Check sheet for the drawn part. Datum: minimum x, y, z corner. Units: mm. Round coordinates to 2 decimals unless told otherwise and drop trailing zeros. Write each loop counter-clockwise with the first axis right and the second up, starting at its lowest first coordinate (ties: lowest second). Pieces come first, ordered by that corner, then holes.
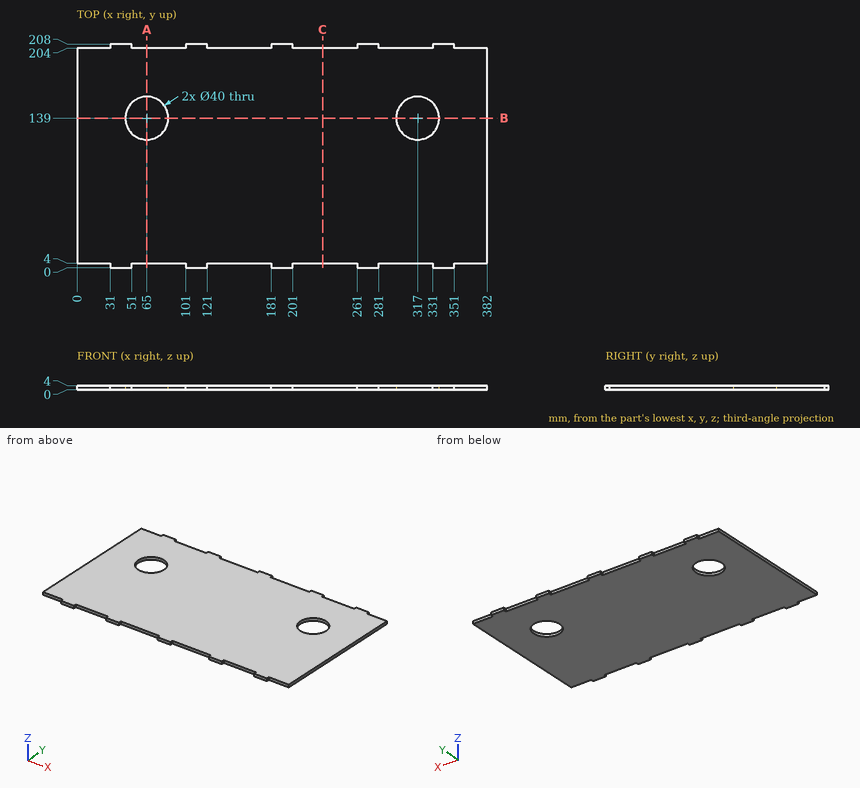
Q1. Sectioned sample at C-C (x = 228.5). Enter the section's corners in (y, z), plus the area to 3 significant figures.
Recorded:
outline: (4, 0) - (204, 0) - (204, 4) - (4, 4) - close
area: 800 mm2
Q2. Sectioned sample at A-A (x = 65). Enter the section's corners in (y, z), plus the area to 3 significant figures.
Recorded:
outline: (4, 0) - (119, 0) - (119, 4) - (4, 4) - close; (159, 0) - (204, 0) - (204, 4) - (159, 4) - close
area: 640 mm2
Q3. Depth check by flat-ended pin: P1, Ø1.2, axis at x = 370.5, z = 1.5, coming from the +Y side; P2, Ø2, axis at x = 305, z = 2, coming from the -Y side; P3, Ø1.2, axis at y = 2.5, z = 2, coming from the +X side. Enter the tip coordinate at first touch or a pass-through.
Recorded:
P1: stops at y = 204
P2: stops at y = 4
P3: stops at x = 351
Q4. Material ranges on line 1 along Y through (x, z) = (317, 2.05); line 2 along Y through (x, z) = (22, 1.1), recorded low to high.
Recorded:
line 1: y = 4 to 119, 159 to 204
line 2: y = 4 to 204
Q5. Sectioned sample at B-B (y = 139). Enter the section's corners in (x, z).
Recorded:
outline: (0, 0) - (45, 0) - (45, 4) - (0, 4) - close; (85, 0) - (297, 0) - (297, 4) - (85, 4) - close; (337, 0) - (382, 0) - (382, 4) - (337, 4) - close
